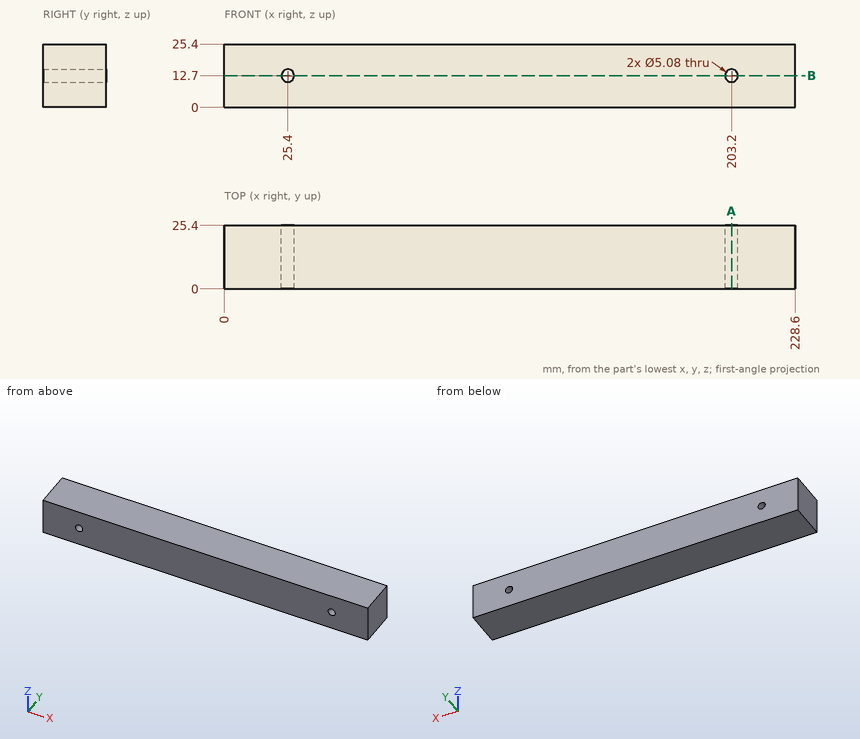
Can you work these out from the drawing? Everything is in mm from the part's minimum corner. Round coordinates to 2 decimals unless told otherwise and drop trailing zeros. Loops run counter-clockwise (first coordinate to the right, second up) from the corner with the lowest first, then second, coordinate; pieces in that order, holes last. Notation, with made-up numbers: M -29,87 L 26,87 A11 ccw 26,103 Z; hole C 22,1.25 d4. An arc over 180 degrees is marked long. Answer in a Markdown table with one row per item.
1. If we section it at A-A, the plane x = 203.2: Please give me the cut outline in (y, z).
Established:
| item | result |
|---|---|
| outline | M 0,0 L 25.4,0 L 25.4,10.16 L 0,10.16 Z; M 0,15.24 L 25.4,15.24 L 25.4,25.4 L 0,25.4 Z |
2. If we section it at B-B, the plane z = 12.7: Please give me the cut outline in (x, y), plus the area to 3 significant figures.
Established:
| item | result |
|---|---|
| outline | M 0,0 L 22.86,0 L 22.86,25.4 L 0,25.4 Z; M 27.94,0 L 200.66,0 L 200.66,25.4 L 27.94,25.4 Z; M 205.74,0 L 228.6,0 L 228.6,25.4 L 205.74,25.4 Z |
| area | 5,550 mm² |
3. I'm going to push a flat-ended pin straight in: pin 1 Ø4 at (x, z) = (25.4, 12.7) entering from -Y. Where does the tip first touch, or does it pass through?
Established:
| item | result |
|---|---|
| pin 1 | through |
4. Please list where these lines run through material, in increasing order: line 1 (X direction, y = 7.75, z = 13.75); line 2 (X direction, y = 21.5, z = 14.75); line 3 (Z direction, x = 25.4, y = 15.25). Write a range as from..to.
Established:
| item | result |
|---|---|
| line 1 | 0..23.09, 27.71..200.89, 205.51..228.6 |
| line 2 | 0..23.9, 26.9..201.7, 204.7..228.6 |
| line 3 | 0..10.16, 15.24..25.4 |
